```python
from build123d import *

# Parameters (mm, degrees)
SKETCH1_R     = 10
SKETCH1_R_2   = 4.5
BODY_DEPTH    = 18.7
CHAMFER1_SIZE = 0.5


with BuildPart() as part:
    # Sketch1 → Body (new body)
    with BuildSketch(Plane(origin=(0, 0, 0), x_dir=(1, 0, 0), z_dir=(0, 1, 0))):
        with Locations(Location((0, 0, 0), (0, 0, 270))):
            Circle(SKETCH1_R)
        with Locations(Location((0, 0, 0), (0, 0, 270))):
            Circle(SKETCH1_R_2, mode=Mode.SUBTRACT)
    extrude(amount=BODY_DEPTH)

    # Chamfer1
    chamfer1_edges = [part.edges().sort_by_distance(p)[0] for p in [
        (0, 0, -10),
        (0, 18.7, -10),
        (0, 0, -4.5),
        (0, 18.7, -4.5),
    ]]
    chamfer(chamfer1_edges, length=CHAMFER1_SIZE)


solid = part.part
```
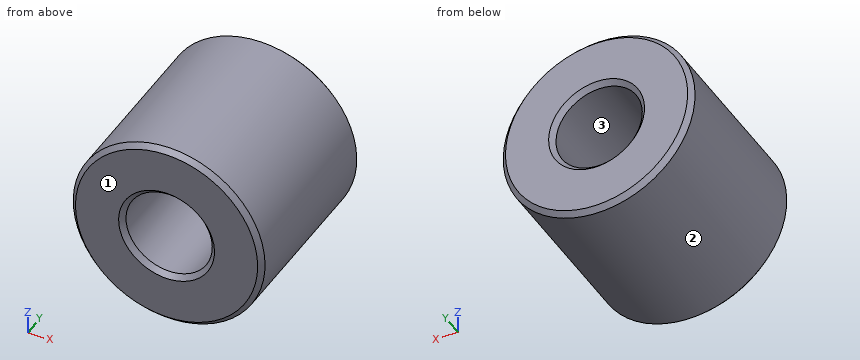
Source: CAD feature listing. Evaluate the final solid. Frame: model axes, mm. Face numbers are marked on the shaded views. Give positions to 0.01 mm unless a question says otherwise; leave off trailing zeros. Loops run counter-clockwise (first coordinate to the right, second up) from the corner with the lowest first, then second, coordinate; pieces in that order, holes last. Notation, with made-up numbers: (80.25, -10.75) -> (100.25, -10.75) arc R17 ccw to (100.25, 18.25) -> close; hole circle Ø6 at (-21, 54.5). An arc over 180 degrees is marked (long way). Put each result on its own line as item: value. Start each with the question number.
1) Material intervals for probe 1 along X at (y, z) = (9, 0); probe 2 along Z at (x, y) = (1.5, 14.25); probe 3 along X at (y, z) = (9.25, -2.25), sorted ascending.
2) Cut plane B-B (x = 0). Return loops of the section in (y, z).
3) Cut plane A-A (z = 0). Return loops of the section in (x, y), then the cut area to 3 significant figures.
4) Contact query for flat-ended pins moving along their axis: P1, Ø4, axis at y = 12.5, z = 5, coming from the -X side; P2, Ø4, axis at y = 10, z = 6.5, coming from the -X side; P3, Ø1, axis at y = 10, z = 7, coming from the +X side. Output: stop coordinate, or through.
5) Draft query along X for the marked faces 1, 2 and 3. Return one class per face: released by +X, released by -X, zero draft, split by the parting line, or undercut.
6) Cut plane C-C (y = 13.75). Return loops of the section in (x, z), then the cut area to 3 significant figures.
Results are:
1. probe 1: x = -10 to -4.5, 4.5 to 10
1. probe 2: z = -9.89 to -4.24, 4.24 to 9.89
1. probe 3: x = -9.74 to -3.9, 3.9 to 9.74
2. outline: (0, -9.5) -> (0.5, -10) -> (18.2, -10) -> (18.7, -9.5) -> (18.7, -5) -> (18.2, -4.5) -> (0.5, -4.5) -> (0, -5) -> close; (0, 5) -> (0.5, 4.5) -> (18.2, 4.5) -> (18.7, 5) -> (18.7, 9.5) -> (18.2, 10) -> (0.5, 10) -> (0, 9.5) -> close
3. outline: (-10, 0.5) -> (-9.5, 0) -> (-5, 0) -> (-4.5, 0.5) -> (-4.5, 18.2) -> (-5, 18.7) -> (-9.5, 18.7) -> (-10, 18.2) -> close; (4.5, 0.5) -> (5, 0) -> (9.5, 0) -> (10, 0.5) -> (10, 18.2) -> (9.5, 18.7) -> (5, 18.7) -> (4.5, 18.2) -> close
3. area: 205 mm2
4. P1: stops at x = -9.54
4. P2: stops at x = -8.93
4. P3: stops at x = 7.6
5. face 1: zero draft
5. face 2: split by the parting line
5. face 3: undercut
6. outline: circle Ø20 at (0, 0); hole circle Ø9 at (0, 0)
6. area: 251 mm2
